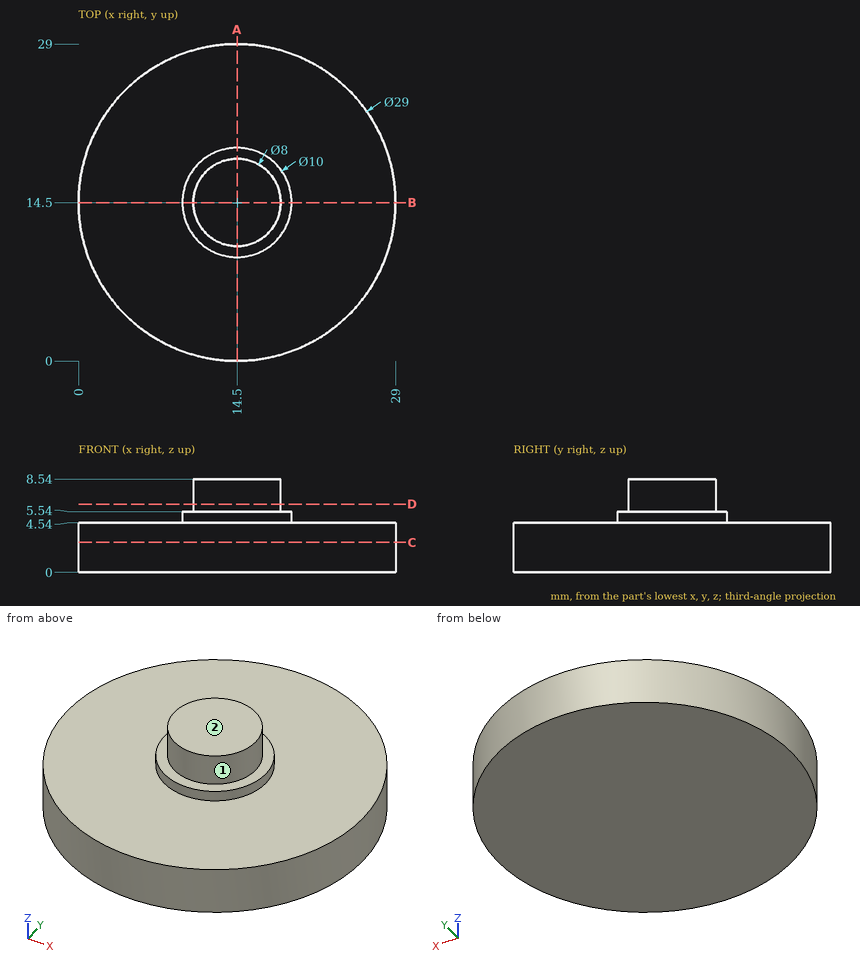
Here's the drawing with two shaded views (mm, measured from the low corner). I have some questions. A direction names the side the tool comes from. Give positions to 0.01 mm unless a question says otherwise; leave off trailing zeros. Write each loop counter-clockwise with the first axis right and the second up, starting at its lowest first coordinate (ties: lowest second). Pieces come first, ordered by that corner, then holes. Notation, with made-up numbers: (21, 79.5) -> (37, 79.5) arc R21 cw to (37, 94.5) -> close; hole circle Ø1 at (-32, 40.25). An arc over 180 degrees is marked (long way). One line per item, written item: value.
Q1. For P1, Ø3, axis at y = 12.5, z = 3.5, coming from the -X side; P2, Ø4, axis at x = 3.5, z = 1, coming from the -Y side; P3, Ø8, axis at x = 8, y = 21, coming from the +Z side, each with a flat end and sliding along its axis, tell me the tip position at first contact or that it passes through.
Results found:
P1: stops at x = 0.01
P2: stops at y = 3.13
P3: stops at z = 4.54
Q2. Imagine slicing it at C-C on z = 2.75. Please give me the cut outline in (x, y).
Results found:
outline: circle Ø29 at (14.5, 14.5)
Q3. Please list where these lines run through material, in increasing order: line 1 (Z direction, x = 2.5, y = 10); line 2 (Y direction, x = 1.75, z = 1.5); line 3 (X direction, y = 13.5, z = 3.25). Write a range as [from, to].
Results found:
line 1: z = [0, 4.54]
line 2: y = [7.59, 21.41]
line 3: x = [0.03, 28.97]
Q4. Imagine slicing it at A-A on x = 14.5. Please give me the cut outline in (y, z).
Results found:
outline: (0, 0) -> (29, 0) -> (29, 4.54) -> (19.5, 4.54) -> (19.5, 5.54) -> (18.5, 5.54) -> (18.5, 8.54) -> (10.5, 8.54) -> (10.5, 5.54) -> (9.5, 5.54) -> (9.5, 4.54) -> (0, 4.54) -> close
Q5. Imagine slicing it at D-D on z = 6.25. Please give me the cut outline in (x, y), and give its area (3 significant figures).
Results found:
outline: circle Ø8 at (14.5, 14.5)
area: 50.3 mm^2
Q6. Which directions (+Z, -Z, +X, -X, +Y, -Y) give clear straight access to the entire face, cutting with the end or side of a thin tool? Please do the marked faces 1 and 2.
Results found:
face 1: +Z
face 2: +Z, +X, -X, +Y, -Y
